from build123d import *

# Parameters (mm, degrees)
SKETCH1_W               = 200
SKETCH1_H               = 80
BOSS_EXTRUDE1_DEPTH     = 10
FILLET1_R               = 5
OTHER_D10_OUTLINE_R     = 2.5
OTHER_D10_OUTLINE_R_2   = 2.25
OTHER_D10_DEPTH         = 10
OTHER_START             = 5
OTHER_D10_2_OUTLINE_R   = 4
OTHER_D10_2_OUTLINE_R_2 = 2.25
OTHER_D10_2_DEPTH       = 5


# Read off the part's stored shape, not the designer's step: the other step
with BuildPart() as part:
    # Sketch1 → Boss-Extrude1 (new body)
    with BuildSketch(Plane(origin=(0, 0, 0), x_dir=(1, 0, 0), z_dir=(0, 1, 0))):
        Rectangle(SKETCH1_W, SKETCH1_H)
    extrude(amount=BOSS_EXTRUDE1_DEPTH)

    # Fillet1
    fillet1_edges = [part.edges().sort_by_distance(p)[0] for p in [
        (-100, 5, -40),
        (100, 5, -40),
        (100, 5, 40),
        (-100, 5, 40),
    ]]
    fillet(fillet1_edges, radius=FILLET1_R)

    # Other D10 outline → Other D10 (cut)
    with BuildSketch(Plane(origin=(0, 0, 0), x_dir=(1, 0, 0), z_dir=(0, 1, 0))):
        with Locations((17.5, 0)):
            Circle(OTHER_D10_OUTLINE_R)
        with Locations((-17.5, 0)):
            Circle(OTHER_D10_OUTLINE_R)
        with Locations((-19, -19)):
            Circle(OTHER_D10_OUTLINE_R)
        with Locations((19, -19)):
            Circle(OTHER_D10_OUTLINE_R)
        with Locations((19, 19)):
            Circle(OTHER_D10_OUTLINE_R)
        with Locations((-19, 19)):
            Circle(OTHER_D10_OUTLINE_R)
        with Locations((-86, 0)):
            Circle(OTHER_D10_OUTLINE_R)
        with Locations((86, 0)):
            Circle(OTHER_D10_OUTLINE_R)
        with Locations((51, 0)):
            Circle(OTHER_D10_OUTLINE_R)
        with Locations((-51, 0)):
            Circle(OTHER_D10_OUTLINE_R)
        with Locations((49.5, -19)):
            Circle(OTHER_D10_OUTLINE_R)
        with Locations((49.5, 19)):
            Circle(OTHER_D10_OUTLINE_R)
        with Locations((-49.5, -19)):
            Circle(OTHER_D10_OUTLINE_R)
        with Locations((-49.5, 19)):
            Circle(OTHER_D10_OUTLINE_R)
        with Locations((87.5, -19)):
            Circle(OTHER_D10_OUTLINE_R)
        with Locations((87.5, 19)):
            Circle(OTHER_D10_OUTLINE_R)
        with Locations((-87.5, -19)):
            Circle(OTHER_D10_OUTLINE_R)
        with Locations((-87.5, 19)):
            Circle(OTHER_D10_OUTLINE_R)
        with Locations((-78, -30)):
            Circle(OTHER_D10_OUTLINE_R_2)
        with Locations((-78, 30)):
            Circle(OTHER_D10_OUTLINE_R_2)
        with Locations((78, -30)):
            Circle(OTHER_D10_OUTLINE_R_2)
        with Locations((78, 30)):
            Circle(OTHER_D10_OUTLINE_R_2)
        with Locations((-34.25, -30)):
            Circle(OTHER_D10_OUTLINE_R_2)
        with Locations((34.25, -30)):
            Circle(OTHER_D10_OUTLINE_R_2)
        with Locations((34.25, 30)):
            Circle(OTHER_D10_OUTLINE_R_2)
        with Locations((-34.25, 30)):
            Circle(OTHER_D10_OUTLINE_R_2)
    extrude(amount=OTHER_D10_DEPTH, mode=Mode.SUBTRACT)

    # Other D10 2 outline → Other D10 2 (cut)
    # profile 1 of 8: a face of its own
    with BuildSketch(Plane(origin=(0, 0, 0), x_dir=(1, 0, 0), z_dir=(0, 1, 0)).offset(OTHER_START)):
        with Locations((-78, -30)):
            Circle(OTHER_D10_2_OUTLINE_R)
        with Locations((-78, -30)):
            Circle(OTHER_D10_2_OUTLINE_R_2, mode=Mode.SUBTRACT)
    # profile 2 of 8: a face of its own
    with BuildSketch(Plane(origin=(0, 0, 0), x_dir=(1, 0, 0), z_dir=(0, 1, 0)).offset(OTHER_START)):
        with Locations((-78, 30)):
            Circle(OTHER_D10_2_OUTLINE_R)
        with Locations((-78, 30)):
            Circle(OTHER_D10_2_OUTLINE_R_2, mode=Mode.SUBTRACT)
    # profile 3 of 8: a face of its own
    with BuildSketch(Plane(origin=(0, 0, 0), x_dir=(1, 0, 0), z_dir=(0, 1, 0)).offset(OTHER_START)):
        with Locations((78, -30)):
            Circle(OTHER_D10_2_OUTLINE_R)
        with Locations((78, -30)):
            Circle(OTHER_D10_2_OUTLINE_R_2, mode=Mode.SUBTRACT)
    # profile 4 of 8: a face of its own
    with BuildSketch(Plane(origin=(0, 0, 0), x_dir=(1, 0, 0), z_dir=(0, 1, 0)).offset(OTHER_START)):
        with Locations((78, 30)):
            Circle(OTHER_D10_2_OUTLINE_R)
        with Locations((78, 30)):
            Circle(OTHER_D10_2_OUTLINE_R_2, mode=Mode.SUBTRACT)
    # profile 5 of 8: a face of its own
    with BuildSketch(Plane(origin=(0, 0, 0), x_dir=(1, 0, 0), z_dir=(0, 1, 0)).offset(OTHER_START)):
        with Locations((-34.25, -30)):
            Circle(OTHER_D10_2_OUTLINE_R)
        with Locations((-34.25, -30)):
            Circle(OTHER_D10_2_OUTLINE_R_2, mode=Mode.SUBTRACT)
    # profile 6 of 8: a face of its own
    with BuildSketch(Plane(origin=(0, 0, 0), x_dir=(1, 0, 0), z_dir=(0, 1, 0)).offset(OTHER_START)):
        with Locations((34.25, -30)):
            Circle(OTHER_D10_2_OUTLINE_R)
        with Locations((34.25, -30)):
            Circle(OTHER_D10_2_OUTLINE_R_2, mode=Mode.SUBTRACT)
    # profile 7 of 8: a face of its own
    with BuildSketch(Plane(origin=(0, 0, 0), x_dir=(1, 0, 0), z_dir=(0, 1, 0)).offset(OTHER_START)):
        with Locations((34.25, 30)):
            Circle(OTHER_D10_2_OUTLINE_R)
        with Locations((34.25, 30)):
            Circle(OTHER_D10_2_OUTLINE_R_2, mode=Mode.SUBTRACT)
    # profile 8 of 8: a face of its own
    with BuildSketch(Plane(origin=(0, 0, 0), x_dir=(1, 0, 0), z_dir=(0, 1, 0)).offset(OTHER_START)):
        with Locations((-34.25, 30)):
            Circle(OTHER_D10_2_OUTLINE_R)
        with Locations((-34.25, 30)):
            Circle(OTHER_D10_2_OUTLINE_R_2, mode=Mode.SUBTRACT)
    extrude(amount=OTHER_D10_2_DEPTH, mode=Mode.SUBTRACT)


solid = part.part
Read the model definition and answer for the solid it produces. Units are mm, in the model's axes. A direction names the side the tool comes from. Give positions to 0.01 mm unless a question says otherwise; leave off trailing zeros. Write each loop counter-clockwise with the first axis right and the second up, starting at its lowest first coordinate (ties: lowest second). Pieces come first, ordered by that corner, then holes. Notation, with made-up numbers: M 18.25,-16 L 76.25,-16 A6 cw 76.25,-8 Z; hole C 9,55 d8. An arc over 180 degrees is marked long. One line per item, written item: value. Start each with the question number.
(1) Determine the mould class of faces 3 (the flat face through (80, 5, 32)), 4 (the cylindrical face through (98, 5, 39)), 5 (the flat face through (-1, 0, -1)), 6 (the flat face through (-100, 5, 0)) for opening direction X: pulls with the +X half, pulls with the -X half, needs draft (parallel to the pull), parting line crosses it, or undercut.
(2) Find the intervals of material crossed by line 1 (Z direction, x = -34.25, y = 4); line 2 (X direction, y = 8.25, z = -30); line 3 (X direction, y = 1.8, z = -30), in increasing order.
(3) Find section A-A (z = 19). Determine the outline of the cut face in (x, y), plus the area to 3 significant figures.
(4) Find section B-B (x = 78). Determine the outline of the cut face in (y, z).
(5) A tool of negligible diameter and unlimited length cuts with its end or side. For faces 1 (the cylindrical face through (80.08, 2.46, 30.86)), 2 (the flat face through (-32.5, 5, -28.3)), from which of +Z, -Z, +X, -X, +Y, -Y can it reach the whole face along a straight path? Write none if from no direction.
(6) A flat-ended cylindrical pin translates along its axis: pin 1 Ø5 at (x, z) = (78, 30) entering from +Y. Find the tip coordinate at first contact, or state that the pin passes through.
(7) Find section C-C (y = 2.25). Give the number of separate pieces and of enclosed holes in the cut face, plus the area to 3 significant figures.
Results below:
1. face 3: undercut
1. face 4: pulls with the +X half
1. face 5: needs draft
1. face 6: pulls with the -X half
2. line 1: z = -40 to -32.25, -27.75 to 27.75, 32.25 to 40
2. line 2: x = -100 to -82, -74 to -38.25, -30.25 to 30.25, 38.25 to 74, 82 to 100
2. line 3: x = -100 to -80.25, -75.75 to -36.5, -32 to 32, 36.5 to 75.75, 80.25 to 100
3. outline: M -100,0 L -90,0 L -90,10 L -100,10 Z; M -85,0 L -52,0 L -52,10 L -85,10 Z; M -47,0 L -21.5,0 L -21.5,10 L -47,10 Z; M -16.5,0 L 16.5,0 L 16.5,10 L -16.5,10 Z; M 21.5,0 L 47,0 L 47,10 L 21.5,10 Z; M 52,0 L 85,0 L 85,10 L 52,10 Z; M 90,0 L 100,0 L 100,10 L 90,10 Z
3. area: 1,700 mm^2
4. outline: M 0,-40 L 10,-40 L 10,-34 L 5,-34 L 5,-32.25 L 0,-32.25 Z; M 0,-27.75 L 5,-27.75 L 5,-26 L 10,-26 L 10,26 L 5,26 L 5,27.75 L 0,27.75 Z; M 0,32.25 L 5,32.25 L 5,34 L 10,34 L 10,40 L 0,40 Z
5. face 1: +Y, -Y
5. face 2: +Y
6. pin 1: stops at y = 5
7. separate pieces: 1
7. enclosed holes: 26
7. area: 15,500 mm^2
